The listing builds one solid part. Answer for the finished solid, in the listing's coordinates (mm). A direction names the side the tool comes from. Give positions to 0.01 mm unless a question says otherwise; leave off trailing zeros. Write each loop counter-clockwise with the first axis right and the second up, starting at its lowest first coordinate (ties: lowest second). Pieces come first, ordered by that corner, then holes. Notation, with made-up numbers: (-34, 48.25) -> (17, 48.25) arc R18 cw to (17, 79.25) -> close; hole circle Ø2 at (-33, -33.75). An arc over 180 degrees is marked (long way). One line per question, with ' | ' between items.
Autodesk Inventor part; units mm, degrees
ref_plane "YZ Plane" through (0, 0, 0) normal (1, 0, 0) x (0, 1, 0)
ref_plane "XZ Plane" through (0, 0, 0) normal (0, 1, 0) x (-1, 0, 0)
ref_plane "XY Plane" through (0, 0, 0) normal (0, 0, 1) x (1, 0, 0)
sketch "Sketch1" plane through (0, 0, 0) normal (0, 0, 1) x (1, 0, 0)
  line L0 (-44.323, 14.2875) -> (44.323, 14.2875)
  line L1 (44.323, 14.2875) -> (44.323, -14.2875)
  line L2 (44.323, -14.2875) -> (-44.323, -14.2875)
  line L3 (-44.323, -14.2875) -> (-44.323, 14.2875)
  point P0 (0, 0)
  dimension "d0" = 88.646
  dimension "d1" = 44.323
  dimension "d2" = 14.2875
  dimension "d3" = 28.575
extrude "Extrusion1" add sketch "Sketch1" along normal mid plane 6.35
sketch "Sketch2" plane through (0, 0, 3.175) normal (0, 0, 1) x (1, 0, 0)
  circle A0 centre (-26.924, 0) radius 11.303
  circle A1 centre (0, 0) radius 11.303
  line L0 (44.323, -14.2875) -> (44.323, 14.2875)
  circle A2 centre (26.924, 0) radius 11.303
  line L1 (-44.323, 14.2875) -> (-44.323, -14.2875)
  line L2 (-44.323, 0) -> (44.323, 0) construction
  line L3 (44.323, 14.2875) -> (-44.323, 14.2875)
  point P0 (0, 0)
  dimension "d6" = 22.606
  dimension "d9" = 22.606
  dimension "d11" = 22.606
  dimension "d14" = 26.924
  dimension "d21" = 88.646
  dimension "d22" = 26.924
  dimension "d45" = 0
sketch "Sketch4" plane through (-44.323, -14.2875, -3.175) normal (-1, 0, 0) x (0, 0, 1)
  line L0 (0, 0) -> (0, 28.575)
  line L1 (6.35, 28.575) -> (6.35, 0)
  line L2 (0, 22.6695) -> (6.35, 22.6695)
  line L3 (6.35, 22.6695) -> (6.35, 5.9055)
  line L4 (6.35, 5.9055) -> (0, 5.9055)
  line L5 (0, 5.9055) -> (0, 22.6695)
  point P0 (3.175, 14.2875)
  dimension "d30" = 8.382
  dimension "d31" = 16.764
extrude "Extrusion3" cut sketch "Sketch4" against normal blind 0.635
mirror "Mirror1" about plane through (0, 0, 0) normal (1, 0, 0) of "Extrusion3"
sketch "Sketch11" plane through (0, 0, -3.175) normal (0, 0, -1) x (-1, 0, 0)
  circle A0 centre (-39.751, 9.7155) radius 3.175
  line L0 (-44.323, 14.2875) -> (-44.323, 8.382)
  line L1 (44.323, 14.2875) -> (-44.323, 14.2875)
  point P0 (0, 0)
  dimension "d72" = 4.572
  dimension "d73" = 4.572
  dimension "d74" = 6.35
extrude "Extrusion10" cut sketch "Sketch11" against normal blind 1.27
sketch "Sketch7" plane through (-44.323, -14.2875, 3.175) normal (0, -1, 0) x (1, 0, 0)
  line L0 (30.353, -14.605) -> (58.293, -14.605)
  line L1 (58.293, -14.605) -> (58.293, 8.255)
  line L2 (58.293, 8.255) -> (30.353, 8.255)
  line L3 (30.353, 8.255) -> (30.353, -14.605)
  point P0 (44.323, -3.175)
  dimension "d39" = 27.94
  dimension "d40" = 22.86
  dimension "d41" = 11.43
  dimension "d42" = 13.97
extrude "Extrusion5" [suppressed]
extrude "Extrusion6" cut sketch "Sketch2" against normal blind 25.4
sketch "Sketch8" plane through (0, 0, -3.175) normal (0, 0, -1) x (-1, 0, 0)
  line L0 (43.688, 8.382) -> (43.688, -8.382) construction
  line L1 (43.688, 0) -> (-43.688, 0)
  line L2 (-43.688, 8.382) -> (-43.688, -8.382) construction
  line L3 (44.323, 14.2875) -> (-44.323, 14.2875)
  line L4 (44.323, 8.382) -> (44.323, 14.2875)
  line L5 (-44.323, 14.2875) -> (-44.323, 8.382)
  line L6 (-43.688, 8.382) -> (-43.688, 0)
  line L7 (-44.323, 8.382) -> (-43.688, 8.382)
  line L8 (43.688, 8.382) -> (43.688, 0)
  line L9 (43.688, 8.382) -> (44.323, 8.382)
  point P0 (0, 0)
extrude "Extrusion7" [suppressed]
sketch "Sketch9" plane through (0, 0, -3.175) normal (0, 0, -1) x (-1, 0, 0)
  line L0 (-44.323, -14.2875) -> (44.323, -14.2875)
  line L1 (44.323, -14.2875) -> (44.323, -8.382)
  line L2 (44.323, -8.382) -> (43.688, -8.382)
  line L3 (-43.688, -8.382) -> (-44.323, -8.382)
  line L4 (-44.323, -8.382) -> (-44.323, -14.2875)
  line L5 (-43.688, 8.382) -> (-43.688, -8.382)
  line L6 (-43.688, 0) -> (-43.688, -8.382)
  line L7 (-43.688, 0) -> (43.688, 0)
  line L8 (43.688, -8.382) -> (43.688, 8.382)
  line L9 (43.688, -8.382) -> (43.688, 0)
  point P0 (0, 0)
extrude "Extrusion8" cut sketch "Sketch9" against normal through all
sketch "Sketch10" plane through (-43.688, 0, -3.175) normal (0, -1, 0) x (1, 0, 0)
  line L0 (5.461, 6.35) -> (5.461, 0)
  line L1 (0, 0) -> (0, 6.35)
  line L2 (-0.635, 0) -> (-0.635, 6.35)
  line L3 (5.461, 6.35) -> (5.461, 0)
  line L4 (0, 6.35) -> (5.461, 6.35)
  line L5 (0, 0) -> (0, 6.35)
  line L6 (5.461, 0) -> (0, 0)
  circle A0 centre (2.7305, 3.81) radius 1.5494
  line L7 (86.614, 1.27) -> (80.264, 1.27)
  line L8 (86.614, 0) -> (80.264, 0)
  point P0 (43.688, 3.175)
  point P1 (84.328, 1.27)
  point P2 (77.978, 1.27)
  point P3 (84.328, 0)
  point P4 (77.978, 0)
  dimension "d58" = 3.0988
  dimension "d61" = 5.461
  dimension "d62" = 2.7305
  dimension "d77" = 5.08
  dimension "d78" = 2.54
extrude "Extrusion9" cut sketch "Sketch10" against normal blind 11.43 contours A0
mirror "Mirror2" about plane through (0, 0, 0) normal (1, 0, 0) of "Extrusion9"
thread "Thread1"
thread "Thread2"
fillet "Fillet1" radius 3.175 2 edges at (-44.323, 14.2875, 0) (44.323, 14.2875, 0)
sketch "Sketch12" plane through (-41.148, 14.2875, -3.175) normal (0, 1, 0) x (1, 0, 0)
  line L0 (82.296, -6.35) -> (0, -6.35)
  line L1 (34.798, 0) -> (47.498, 0)
  line L2 (47.498, 0) -> (47.498, -6.35)
  line L3 (47.498, -6.35) -> (34.798, -6.35)
  line L4 (34.798, -6.35) -> (34.798, 0)
  circle A0 centre (41.148, -3.175) radius 1
  line L5 (29.845, 0) -> (52.451, 0)
  dimension "d81" = 6.35
  dimension "d82" = 12.7
  dimension "d83" = 2
  dimension "d87" = 0
extrude "Extrusion11" add sketch "Sketch12" along normal blind 3.8
fillet "Fillet3" radius 3.175 2 edges at (6.35, 14.2875, 0) (-6.35, 14.2875, 0)
equation "\"d9\" = d7"
equation "\"d11\" = d9"
equation "\"d22\" = d14"
equation "\"d62\" = 0.5 * d61"
equation "\"d78\" = 0.5 * d77"
equation "\"d7\" = d6"
properties part number "Tube Holder Halve 2" material "Aluminum 6061-AHC"
Item 1: Determine the mould class of faces 4 (the face through (-1, 13, -3.175)), 5 (the face through (-7.3, 15.2, 0)), 6 (the face through (-26.7, 11.3, 0)), 7 (the face through (36.82, 8.5, -2.55)) for opening direction Y: pulls with the +Y half, pulls with the -Y half, needs draft (parallel to the pull), parting line crosses it, or undercut.
Answers below:
face 4: needs draft | face 5: pulls with the +Y half | face 6: pulls with the -Y half | face 7: undercut
Item 2: Find section B-B (y = 4.75). Write down the section's boundary in (x, z) (1 decimal).
Answers below:
outline: (-43.7, -3.2) -> (-37.2, -3.2) -> (-37.2, 3.2) -> (-43.7, 3.2) -> close; (-16.7, -3.2) -> (-10.3, -3.2) -> (-10.3, 3.2) -> (-16.7, 3.2) -> close; (10.3, -3.2) -> (16.7, -3.2) -> (16.7, 3.2) -> (10.3, 3.2) -> close; (37.2, -3.2) -> (43.7, -3.2) -> (43.7, 3.2) -> (37.2, 3.2) -> close; hole circle Ø3.1 at (-41, 0.6); hole circle Ø3.1 at (41, 0.6)
Item 3: A tool of negligible diameter and unlimited length cuts with its end or side. For faces 1 (the face through (0, 16, -1)), 2 (the face through (25, 14.288, 0)), 3 (the face through (40, 10, -1.905)), from which of +Z, -Z, +X, -X, +Y, -Y can it reach the whole face along a straight path? Write none if from no direction.
Answers below:
face 1: +Y | face 2: +Z, -Z, +X, +Y | face 3: -Z
Item 4: Flat-ended cylindrical pins translate along their axes: pin 1 (3 mm diameter, centred on y = 2.5, z = -0.5, fed in from +X); pin 2 (4 mm diameter, centred on x = 39.75, y = 9.72, fed in from -Z) (3 decimals); pin 3 (1 mm diameter, centred on y = 7.5, z = 2.5, fed in from -X). Find the tip coordinate at first contact, or state that the pin passes through.
Answers below:
pin 1: x = 43.69 | pin 2: z = -1.905 | pin 3: x = -43.69
Item 5: Consider line 1 (Z direction, x = 0, y = 16.1) (3 decimals); line 2 (X direction, y = 2, z = -1.5); line 3 (X direction, y = 7.25, z = 0.25). Determine where each line is inside the solid, lowest interval first. Write a range as [from, to].
Answers below:
line 1: [-3.175, -1], [1, 3.175] | line 2: [-43.69, -38.05], [-15.8, -11.12], [11.12, 15.8], [38.05, 43.69] | line 3: [-43.69, -42.46], [-39.46, -35.6], [-18.25, -8.67], [8.67, 18.25], [35.6, 39.46], [42.46, 43.69]
Item 6: Find section A-A (x = 0). Write down the section's boundary in (y, z) (1 decimal), then the cut area to 3 significant figures.
Answers below:
outline: (11.3, -3.2) -> (18.1, -3.2) -> (18.1, -1) -> (14.3, -1) -> (14.3, 1) -> (18.1, 1) -> (18.1, 3.2) -> (11.3, 3.2) -> close | area: 35.5 mm²
Item 7: Find section D-D (x = 25). Write down the section's boundary in (y, z) (1 decimal).
Answers below:
outline: (11.1, -3.2) -> (14.3, -3.2) -> (14.3, 3.2) -> (11.1, 3.2) -> close
Item 8: Find section C-C (x = 14). Write down the section's boundary in (y, z) (1 decimal), then the cut area to 3 significant figures.
Answers below:
outline: (0, -3.2) -> (14.3, -3.2) -> (14.3, 3.2) -> (0, 3.2) -> close | area: 90.7 mm²
